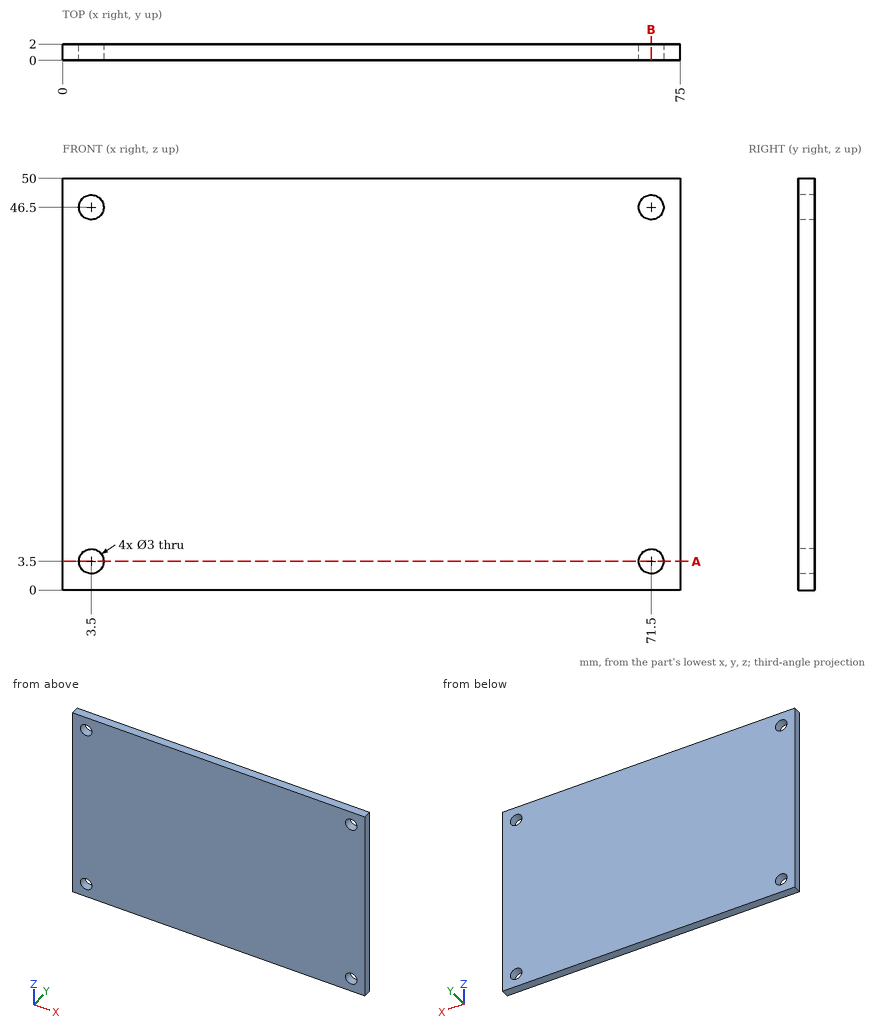
Input: dimensioned drawing with shaded views. Units: mm. Origin: part minimum x, y, z. Round coordinates to 2 decimals unless told otherwise and drop trailing zeros. Loops run counter-clockwise (first coordinate to the right, second up) from the corner with the lowest first, then second, coordinate; pieces in that order, holes last.
1) Material intervals for line 1 (Z direction, x = 3.5, y = 0.85); line 2 (Z direction, x = 4, y = 0.85), sorted ascending.
Ans:
line 1: z = 0 to 2, 5 to 45, 48 to 50
line 2: z = 0 to 2.09, 4.91 to 45.09, 47.91 to 50
2) Pin query (flat end, axial travel): pin 1 (1.8 mm diameter, centred on x = 3.5, z = 3.5, fed in from -Y) (3 decimals). Return the tip coordinate at first contact, or that it passes through.
Ans:
pin 1: passes through
3) Section query A-A on z = 3.5. Return the cut outline in (x, y), plus the area to 3 significant figures.
Ans:
outline: (0, 0) - (2, 0) - (2, 2) - (0, 2) - close; (5, 0) - (70, 0) - (70, 2) - (5, 2) - close; (73, 0) - (75, 0) - (75, 2) - (73, 2) - close
area: 138 mm2
4) Section query B-B on x = 71.5. Return the cut outline in (y, z).
Ans:
outline: (0, 0) - (2, 0) - (2, 2) - (0, 2) - close; (0, 5) - (2, 5) - (2, 45) - (0, 45) - close; (0, 48) - (2, 48) - (2, 50) - (0, 50) - close
